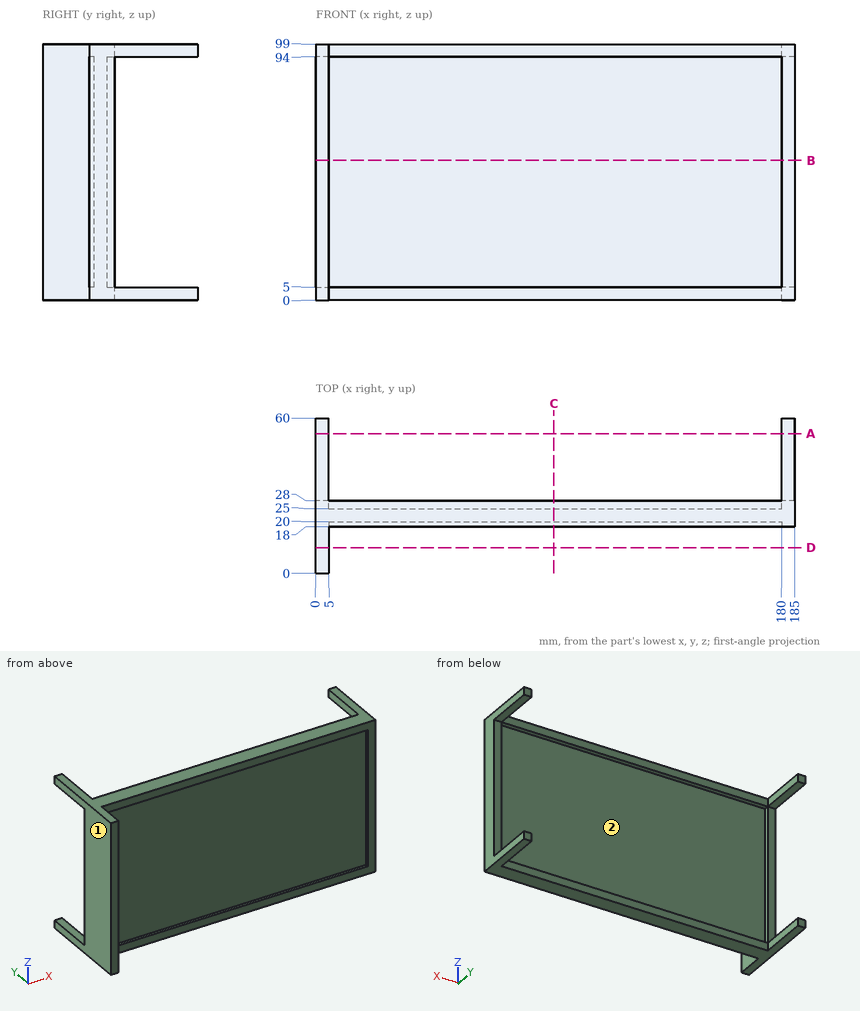
For this review, use the dimensioned drawing (mm, ordinates from the lowest corner) and the shaded views. Round coordinates to 2 decimals unless told otherwise and drop trailing zeros. Order: outer loops, then holes, each group sorted by start corner. A loop starts at its lowest first (then second) coordinate and runs counter-clockwise, first axis right, second up. Notation, with made-up numbers: (34.25, 0.5) -> (84.25, 0.5) arc R8 cw to (84.25, 9.5) -> close; hole circle Ø7 at (11.5, -34.5). An arc over 180 degrees is marked (long way). Use CSV: the item, a comma, the result in double quotes. Start each with the question number.
(1) Consider section C-C on x = 92. Write out the cut boundary in (y, z), and give its area (3 significant figures).
(2) Wall thickness on probe 1 along Z at (x, y) = (41, 19); probe 2 along X at (y, z) = (26.5, 31.5); probe 3 along Y at (x, z) = (133, 43): over which ranges is each line inside the solid? List them lowest first. Write a range as from..to.
(3) Consider section D-D on y = 10. Write out the cut boundary in (x, z), and give its area (3 significant figures).
(4) Consider section A-A on y = 54. Write out the cut boundary in (x, z).
(5) Mouldability with a two-part tool opening along X and no side actions: class the marked faces 1 and 2 as pulls with the +X half, pulls with the -X half, needs draft (parallel to the pull), parting line crosses it, or undercut.
(6) Insertion check: pin 1 (1.5 mm diameter, centred on x = 1.5, z = 39, fed in from +Y); pin 2 (10 mm diameter, centred on x = 101, y = 8.5, fed in from -Z); pin 3 (6 mm diameter, centred on x = 128, z = 21, fed in from -Y); pin 4 (10 mm diameter, centred on y = 10, z = 25, fed in from +X). Each pin has a flat end and moves straight along its axis. Give the tip position at first contact, or say it passes through.
(7) Consider section B-B on z = 54. Write out the cut boundary in (x, y), and give its area (4 significant figures).
Responses:
1,outline,"(18, 0) -> (28, 0) -> (28, 5) -> (25, 5) -> (25, 94) -> (28, 94) -> (28, 99) -> (18, 99) -> (18, 94) -> (20, 94) -> (20, 5) -> (18, 5) -> close"
1,area,"545 mm²"
2,probe 1,"0..5, 94..99"
2,probe 2,"0..5, 180..185"
2,probe 3,"20..25"
3,outline,"(0, 0) -> (5, 0) -> (5, 99) -> (0, 99) -> close"
3,area,"495 mm²"
4,outline,"(0, 0) -> (5, 0) -> (5, 5) -> (0, 5) -> close; (0, 94) -> (5, 94) -> (5, 99) -> (0, 99) -> close; (180, 0) -> (185, 0) -> (185, 5) -> (180, 5) -> close; (180, 94) -> (185, 94) -> (185, 99) -> (180, 99) -> close"
5,face 1,"pulls with the -X half"
5,face 2,"undercut"
6,pin 1,"y = 28"
6,pin 2,"through"
6,pin 3,"y = 20"
6,pin 4,"x = 5"
7,outline,"(0, 0) -> (5, 0) -> (5, 20) -> (180, 20) -> (180, 18) -> (185, 18) -> (185, 28) -> (180, 28) -> (180, 25) -> (5, 25) -> (5, 28) -> (0, 28) -> close"
7,area,"1,065 mm²"
